Check sheet for the modelled part. Datum: model origin and axes. Units: mm. A direction names the side the tool comes from. Coordinates: 2 decimals unless noted, no trailing zeros. Loops run counter-clockwise (first coordinate to the right, second up) from the corner with the lowest first, then second, coordinate; pieces in that order, holes last. Notation, with made-up numbers: M 52,23.25 L 67,23.25 A32 ccw 67,58.25 Z; hole C 15,84 d7. An arc over 180 degrees is marked long. Return JSON: item names as keys, results as strings.
from build123d import *

# Parameters (mm, degrees)
F0_W      = 200
F0_H      = 150
F1_DEPTH  = 2
F2_W      = 5
F2_H      = 5
F2_W_2    = 190
F2_H_2    = 145
F3_DEPTH  = 100
F4_W      = 2
F4_H      = 2
F5_DEPTH  = 90
F7_W      = 2
F7_H      = 2
F8_DEPTH  = 2
F10_W     = 2
F10_H     = 2
F11_DEPTH = 2
F13_W     = 2
F13_H     = 2
F14_DEPTH = 2
F16_W     = 102
F16_H     = 30
F17_DEPTH = 2


with BuildPart() as f1:
    # F0 (on Top) → F1 (new body)
    with BuildSketch(Plane.XY):
        Rectangle(F0_W, F0_H)
    extrude(amount=F1_DEPTH)

    # F2 (on face) → F3 (join)
    with BuildSketch(Plane.XY.offset(2)):
        with Locations((-97.5, 72.5)):
            Rectangle(F2_W, F2_H)
        with Locations((0, 72.5)):
            Rectangle(F2_W_2, F2_H)
        with Locations((-97.5, -2.5)):
            Rectangle(F2_W, F2_H_2)
        with Locations((97.5, 72.5)):
            Rectangle(F2_W, F2_H)
        with Locations((97.5, -2.5)):
            Rectangle(F2_W, F2_H_2)
    extrude(amount=F3_DEPTH)

    # F4 (on face) → F5 (join)
    with BuildSketch(Plane.XY.offset(2)):
        with Locations((93, 68)):
            Rectangle(F4_W, F4_H)
        with Locations((-7, 68)):
            Rectangle(F4_W, F4_H)
        with Locations((-7, 40)):
            Rectangle(F4_W, F4_H)
        with Locations((93, 40)):
            Rectangle(F4_W, F4_H)
        with Locations((-92, 67)):
            Rectangle(F4_W, F4_H)
        with Locations((-92, -15)):
            Rectangle(F4_W, F4_H)
        with Locations((-77, 67)):
            Rectangle(F4_W, F4_H)
        with Locations((-75, -15)):
            Rectangle(F4_W, F4_H)
    extrude(amount=F5_DEPTH)

    # F7 (on offset) → F8 (join)
    with BuildSketch(Plane.XY.offset(82)):
        with Locations((-7, 40)):
            Rectangle(F7_W, F7_H)
        Polygon((-8, 69), (-8, 41), (-6, 41), (-6, 39), (94, 39), (94, 67), (92, 67), (92, 69), align=None)
        with Locations((93, 68)):
            Rectangle(F7_W, F7_H)
    extrude(amount=F8_DEPTH)

    # F10 (on offset) → F11 (join)
    with BuildSketch(Plane.XY.offset(4)):
        Polygon((92, 41), (94, 41), (94, 67), (92, 67), (92, 69), (-6, 69), (-6, 67), (-8, 67), (-8, 41), (-6, 41), (-6, 39), (92, 39), align=None)
        with Locations((93, 40)):
            Rectangle(F10_W, F10_H)
        with Locations((93, 68)):
            Rectangle(F10_W, F10_H)
        with Locations((-7, 40)):
            Rectangle(F10_W, F10_H)
        with Locations((-7, 68)):
            Rectangle(F10_W, F10_H)
    extrude(amount=F11_DEPTH)

    # F13 (on offset) → F14 (join)
    with BuildSketch(Plane.XY.offset(31)):
        Polygon((92, 41), (94, 41), (94, 67), (92, 67), (92, 69), (-6, 69), (-6, 67), (-8, 67), (-8, 41), (-6, 41), (-6, 39), (92, 39), align=None)
        with Locations((93, 40)):
            Rectangle(F13_W, F13_H)
        with Locations((93, 68)):
            Rectangle(F13_W, F13_H)
        with Locations((-7, 40)):
            Rectangle(F13_W, F13_H)
        with Locations((-7, 68)):
            Rectangle(F13_W, F13_H)
    extrude(amount=F14_DEPTH)

    # F16 (on offset) → F17 (join)
    with BuildSketch(Plane.XY.offset(58)):
        with Locations((43, 54)):
            Rectangle(F16_W, F16_H)
    extrude(amount=F17_DEPTH)


solid = f1.part
1) Section check D-D on z = 9.5. Count the separate pieces of the cut face and the enclosed holes in it, then the cut area to 3 significant figures.
Answers:
{"separate pieces": "9", "enclosed holes": "0", "area": "2,480 mm²"}
2) Section check B-B on y = 33. Record the cut outline in (x, z).
Answers:
{"outline": "M -100,0 L 100,0 L 100,102 L 95,102 L 95,2 L -95,2 L -95,102 L -100,102 Z"}
3) Section check C-C on x = -59.5. Record the cut outline in (y, z).
Answers:
{"outline": "M -75,0 L 75,0 L 75,102 L 70,102 L 70,2 L -75,2 Z"}
4) Go/stop test with flat-tipped pins: pin 1 Ø1.6 at (x, z) = (93, 44) entering from -Y; pin 2 Ø1.5 at (x, y) = (-45, 5) entering from +Z; pin 3 Ø3 at (x, y) = (46.5, -7.5) entering from -Z; pin 4 Ø1 at (x, z) = (-75, 34.5) entering from -Y. Record where each tip stops, or that it passes through.
Answers:
{"pin 1": "y = 39", "pin 2": "z = 2", "pin 3": "z = 0", "pin 4": "y = -16"}
5) Scan lines: line 1 along Y through (x, z) = (-91.5, 39); line 2 along Z through (x, y) = (69, 50); line 3 along X through (y, z) = (0, 55). Record each from-to range of solid material in increasing order. Write a range as [from, to].
Answers:
{"line 1": "[-16, -14], [66, 68], [70, 75]", "line 2": "[0, 2], [4, 6], [31, 33], [58, 60], [82, 84]", "line 3": "[-100, -95], [95, 100]"}
6) Set-up check for faces 4 (the face through (100, -1, 50)), 5 (the face through (94, 40.6, 56.8)): record each of +Z, -Z, +X, -X, +Y, -Y from which the full face is reachable in a straight line by a thin tool's end or side.
Answers:
{"face 4": "+Z, -Z, +X, +Y, -Y", "face 5": "+Z, -Y"}
7) Section check A-A on x = 33.5. Record the cut outline in (y, z).
Answers:
{"outline": "M -75,0 L 75,0 L 75,102 L 70,102 L 70,2 L -75,2 Z; M 39,4 L 69,4 L 69,6 L 39,6 Z; M 39,31 L 69,31 L 69,33 L 39,33 Z; M 39,58 L 69,58 L 69,60 L 39,60 Z; M 39,82 L 69,82 L 69,84 L 39,84 Z"}
8) Draft check along Y on faces 1 (the face through (95, -4, 51)), 2 (the face through (20, 69, 83)), 3 (the face through (1, 75, 50)). Enter one of: +Y half, -Y half, draft (parallel to the pull), parting line (faces both ways), or undercut.
Answers:
{"face 1": "draft", "face 2": "undercut", "face 3": "+Y half"}
